Answer from the drawing. Dimensions are ordinates in mm from the lowest x, y and z of the part. Coordinates: 2 decimals unless noted, no trailing zeros. Order: outer loops, then holes, each group sorted by start corner. A loop starts at its lowest first (then second) coordinate and runs counter-clockwise, first axis right, second up. Notation, with made-up numbers: (-34, 4) - (-28, 4) arc R9 cw to (-28, 19) - close; hole circle Ø10 at (-8, -5.5). An arc over 180 degrees is marked (long way). Use a Markdown table: item, result. Add a question column.
Item 1: The part is cut by section A-A, the plane z = 70. Give the vertices of the cut face in (x, y), then the cut area to 3 significant figures.
Item 2: The mould has two halves that part along X. Classify the marked faces 1, 2 and 3: released by +X, released by -X, zero draft, split by the parting line, or undercut.
Item 3: The part is cut by section D-D, the plane z = 49. Give the vertices of the cut face in (x, y).
Item 4: Find the intervals of material crossed by line 1 along X through (y, z) = (9, 70); line 2 along Y through (x, z) = (19.5, 84); line 3 along Z through (x, y) = (106, 7.25), in increasing order.
Item 5: The part is cut by section C-C, the plane y = 8. Give the vertices of the cut face in (x, z), then the cut area to 3 significant figures.
Item 6: Flat-ended cylindrical pins translate along their axes: P1, Ø1.5, axis at x = 37.5, y = 8.5, coming from the +Z side; P2, Ø2, axis at x = 81.5, z = 123.5, coming from the +Y side; P3, Ø5, axis at y = 1.5, z = 118.5, coming from the +X side. Find the tip coordinate at first contact, or state that the pin passes through.
Item 7: The part is cut by section B-B, the plane x = 70. Give the vertices of the cut face in (y, z).
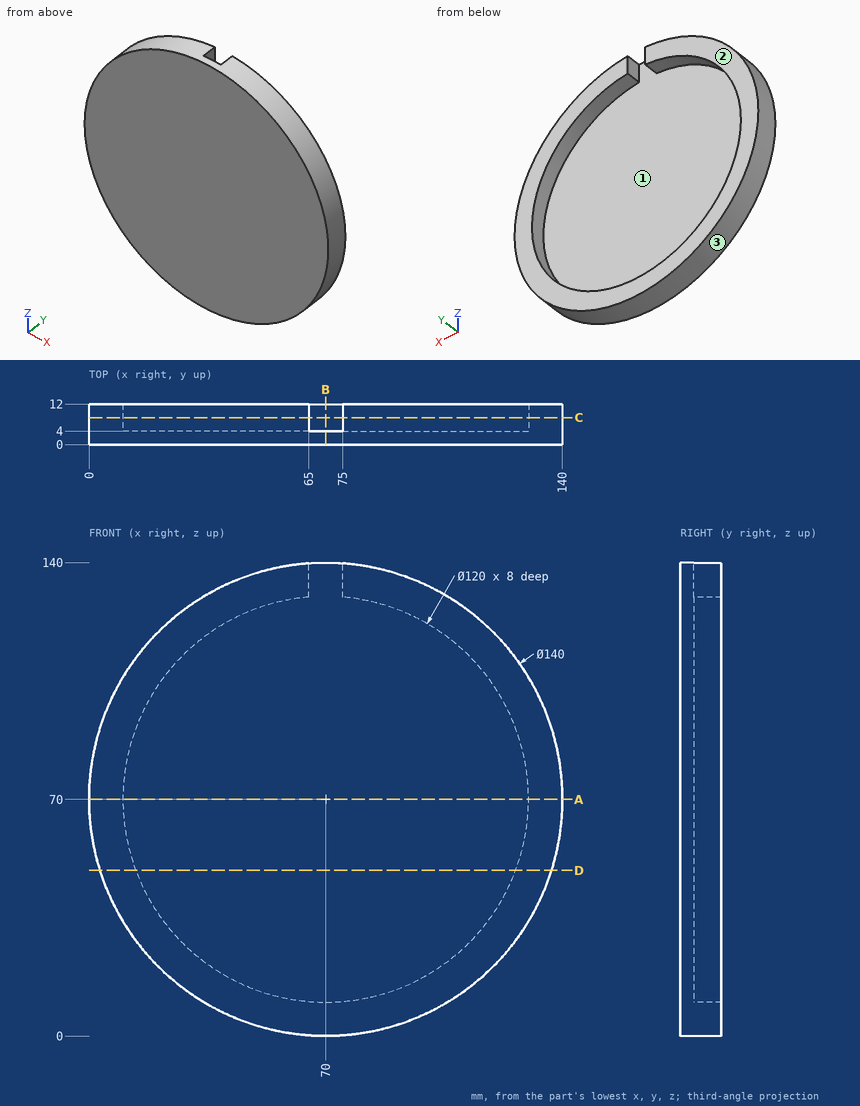
Solution:
| question | item | result |
|---|---|---|
| 1 | outline | (0, 0) - (140, 0) - (140, 12) - (130, 12) - (130, 4) - (10, 4) - (10, 12) - (0, 12) - close |
| 1 | area | 720 mm2 |
| 2 | face 1 | undercut |
| 2 | face 2 | zero draft |
| 2 | face 3 | split by the parting line |
| 3 | outline | (3.22, 0) - (136.78, 0) - (136.78, 12) - (126.2, 12) - (126.2, 4) - (13.8, 4) - (13.8, 12) - (3.22, 12) - close |
| 4 | line 1 | x = 0 to 10, 130 to 140 |
| 4 | line 2 | y = 0 to 4 |
| 4 | line 3 | z = 9.97 to 22, 118 to 130.03 |
| 5 | outline | (65, 129.79) - (65, 139.82) arc R70 ccw (long way) to (75, 139.82) - (75, 129.79) arc R60 cw (long way) to start |
| 5 | area | 3,980 mm2 |
| 6 | P1 | stops at z = 132.39 |
| 6 | P2 | stops at y = 4 |
| 6 | P3 | stops at x = 122.76 |
| 7 | outline | (0, 0) - (12, 0) - (12, 10) - (4, 10) - (4, 140) - (0, 140) - close |
